Input: part model. Units: mm. Frame: model coordinates. Face numbers are marked on the shaded views. Round coordinates to 2 decimals unless told otherwise and drop trailing zeros. Order: outer loops, then holes, each group sorted by start corner. A loop starts at its lowest first (then second) coordinate and runs counter-clockwise, first axis right, second up. Notation, with made-up numbers: (49.5, 87) -> (65.5, 87) arc R9 ccw to (65.5, 102) -> close; hole circle Ø11 at (-32, -14.75). An arc over 180 degrees is marked (long way). Answer as CSV lines item,"result". Start each with the question number.
1) Section query A-A, the plane y = 0. Output: boundary loops of the cut face in (x, z) (3 decimals).
2) Section query D-D, the plane z = 7.5. Output: boundary loops of the cut face in (x, y).
3) Mould query, pull axis X, two halves, no side actions, for the marked faces 1 and 2. Classes: +X half, -X half, draft (parallel to the pull), parting line (faces both ways), or undercut.
4) Section query B-B, the plane z = 5.5. Output: boundary loops of the cut face in (x, y).
5) First-contact query: P1, Ø5, axis at y = -3.5, z = 1.5, coming from the +X side; P2, Ø1, axis at y = -2.5, z = -7.5, coming from the +X side; P3, Ø5, axis at x = -11.5, z = 5.5, coming from the -Y side. Flat tips, straight axial feed; report the tip coordinate or a pass-through.
6) Section query C-C, the plane x = 0. Output: boundary loops of the cut face in (y, z) (3 decimals).
7) Line query: L1, parallel to X at y = 0, z = 5; L2, parallel to X at y = 0, z = 7.25; L3, parallel to Y at x = 0, z = 2.5. Output: solid intervals per line, ascending.
```python
from build123d import *

# Parameters (mm, degrees)
F0_R     = 9.525
F1_DEPTH = 25.019
F2_R     = 9.525
F4_R     = 2.38125
F5_DEPTH = 9.525


with BuildPart() as f1:
    # F0 (on Right) → F1 (new body, symmetric)
    with BuildSketch(Plane.YZ):
        Circle(F0_R)
    extrude(amount=F1_DEPTH, both=True)

    # F2
    f2_edges = [f1.edges().sort_by_distance(p)[0] for p in [
        (-25.019, -9.525, 0),
        (25.019, -9.525, 0),
    ]]
    fillet(f2_edges, radius=F2_R)

    # F4 (on plane+point) → F5 (cut)
    with BuildSketch(Plane.XY.offset(9.525)):
        Circle(F4_R)
    extrude(amount=-F5_DEPTH, mode=Mode.SUBTRACT)


solid = f1.part
```
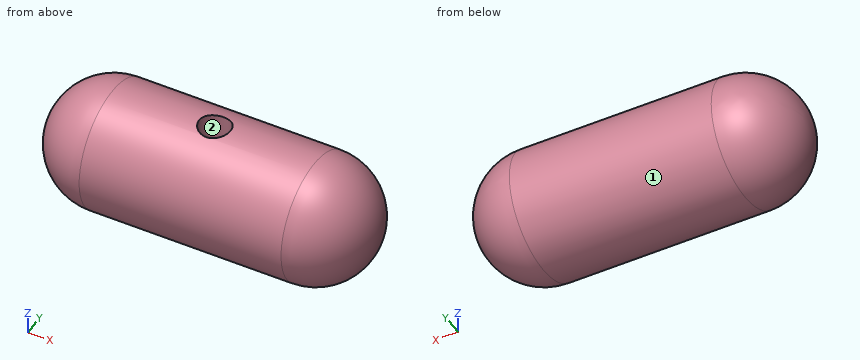
Findings:
1,outline,"(-15.494, -9.525) -> (15.494, -9.525) arc R9.525 ccw to (15.494, 9.525) -> (2.381, 9.525) -> (2.381, 0) -> (-2.381, 0) -> (-2.381, 9.525) -> (-15.494, 9.525) arc R9.525 ccw to start"
2,outline,"(-15.49, -5.87) -> (15.49, -5.87) arc R5.87 ccw to (15.49, 5.87) -> (-15.49, 5.87) arc R5.87 ccw to start; hole circle Ø4.76 at (0, 0)"
3,face 1,"draft"
3,face 2,"undercut"
4,outline,"(-15.49, -7.78) -> (15.49, -7.78) arc R7.78 ccw to (15.49, 7.78) -> (-15.49, 7.78) arc R7.78 ccw to start; hole circle Ø4.76 at (0, 0)"
5,P1,"stops at x = 24.93"
5,P2,"stops at x = 21.48"
5,P3,"stops at y = -9.04"
6,outline,"(-2.381, 0) -> (-2.381, 9.223) arc R9.525 ccw (long way) to (2.381, 9.223) -> (2.381, 0) -> close"
7,L1,"x = -23.6 to -2.38, 2.38 to 23.6"
7,L2,"x = -21.67 to -2.38, 2.38 to 21.67"
7,L3,"y = -9.19 to -2.38, 2.38 to 9.19"
